Source: CAD feature listing. Evaluate the final solid. Frame: model axes, mm. Face numbers are marked on the shaded views. Round coordinates to 2 decimals unless told otherwise and drop trailing zeros. Order: outer loops, then holes, each group sorted by start corner. A loop starts at its lowest first (then second) coordinate and runs counter-clockwise, first axis right, second up. Notation, with made-up numbers: (69.5, 41.25) -> (91.5, 41.25) arc R23 cw to (91.5, 77.25) -> close; hole circle Ø11 at (5.25, 16). An arc over 180 degrees is marked (long way). One line per item, written item: value. Start each with the question number.
1) Mould query, pull axis X, two halves, no side actions, for the marked faces 1, 2, 3 and 4. Classes: pulls with the +X half, pulls with the -X half, needs draft (parallel to the pull), parting line crosses it, or undercut.
2) Section C-C (z = 2.5). Return the cut outline in (x, y), and give its area (3 significant figures).
3) Ray query, L1, parallel to X at y = 1.25, z = 0; L2, parallel to Z at x = 0, y = 1.4; L3, parallel to X at y = 0.4, z = 0.5. Return the intervals inside material, ascending.
4) Section D-D (x = 2.5). Return the cut outline in (y, z), and give its area (3 significant figures).
5) Section A-A (x = 0). Return the cut outline in (y, z).
6) Section B-B (y = 0.8). Return the cut outline in (x, z), and give its area (3 significant figures).
7) Pin query (flat end, axial travel): P1, Ø1.5, axis at x = -4, z = -8.5, coming from the -Y side. Return the tip coordinate at first contact, or that it passes through.
```python
from build123d import *

# Parameters (mm, degrees)
ESQUISSE1_R        = 1
BOSS_EXTRU_1_DEPTH = 2


with BuildPart() as part:
    # Esquisse1 → Boss.-Extru.1 (new body)
    with BuildSketch(Plane(origin=(0, 0, 0), x_dir=(1, 0, 0), z_dir=(0, 1, 0))):
        with BuildLine():
            Line((-6, 0), (-6, 10))
            Line((-6, 10), (9, 10))
            Line((9, 10), (9, -1.732050808))
            Line((9, -1.732050808), (3, -5.196152423))
            ThreePointArc((3, -5.196152423), (-3, -5.196152423), (-6, 0))
        make_face()
        Circle(ESQUISSE1_R, mode=Mode.SUBTRACT)
    extrude(amount=BOSS_EXTRU_1_DEPTH)


solid = part.part
```
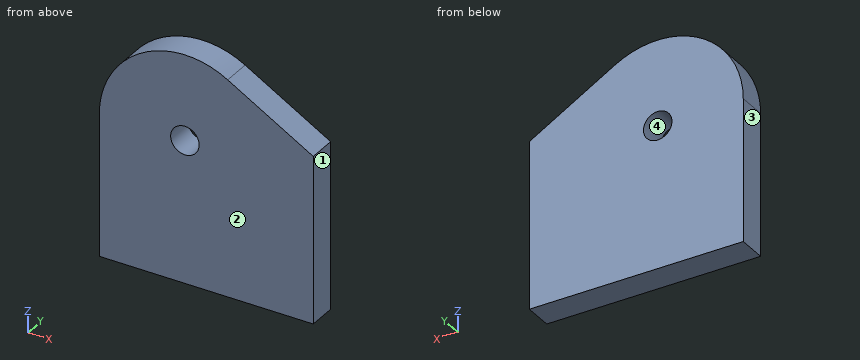
Findings:
1. face 1: pulls with the +X half
1. face 2: needs draft
1. face 3: pulls with the -X half
1. face 4: undercut
2. outline: (-5.45, 0) -> (7.67, 0) -> (7.67, 2) -> (-5.45, 2) -> close
2. area: 26.2 mm2
3. L1: -6 to -1, 1 to 9
3. L2: -10 to -1, 1 to 6
3. L3: -5.98 to -0.87, 0.87 to 9
4. outline: (0, -10) -> (2, -10) -> (2, 5.45) -> (0, 5.45) -> close
4. area: 30.9 mm2
5. outline: (0, -10) -> (2, -10) -> (2, -1) -> (0, -1) -> close; (0, 1) -> (2, 1) -> (2, 6) -> (0, 6) -> close
6. outline: (-6, -10) -> (9, -10) -> (9, 1.73) -> (3, 5.2) arc R6 ccw to (-6, 0) -> close; hole circle Ø2 at (0, 0)
6. area: 213 mm2
7. P1: y = 0
